Can you work these out from the model? Positions are in its coordinate system, mm. A direction names the side the tool comes from. Round coordinates to 2 decimals unless told otherwise and drop trailing zeros.
```python
from build123d import *

# Parameters (mm, degrees)
ESBO_O1_W             = 8
ESBO_O1_H             = 8
CORTE_EXTRUS_O1_DEPTH = 46
ESBO_O3_R             = 2.5
CORTE_EXTRUS_O2_DEPTH = 123.5


with BuildPart() as part:
    # Sketch1 → Revolve1 (revolve)
    with BuildSketch(Plane.XY):
        with BuildLine():
            Line((0, -20), (0, -122))
            ThreePointArc((0, -122), (0.146446609, -122.353553391), (0.5, -122.5))
            Line((0.5, -122.5), (9.616336506, -122.5))
            ThreePointArc((9.616336506, -122.5), (9.920717221, -122.39667667), (10.099299419, -122.129409523))
            Line((10.099299419, -122.129409523), (12.679491924, -112.5))
            Line((12.679491924, -112.5), (22.320508076, -112.5))
            Line((22.320508076, -112.5), (24.900700581, -122.129409523))
            ThreePointArc((24.900700581, -122.129409523), (25.079282779, -122.39667667), (25.383663494, -122.5))
            Line((25.383663494, -122.5), (34.5, -122.5))
            ThreePointArc((34.5, -122.5), (34.853553391, -122.353553391), (35, -122))
            Line((35, -122), (35, -50))
            Line((35, -50), (44.5, -50))
            ThreePointArc((44.5, -50), (44.853553391, -49.853553391), (45, -49.5))
            Line((45, -49.5), (45, -10))
            Line((45, -10), (2.5, -10))
            Line((2.5, -10), (0, -20))
        make_face()
    revolve(axis=Axis((0, 0, 0), (1, 0, 0)))

    # Esboço1 → Corte-extrusão1 (cut, through all)
    with BuildSketch(Plane.ZY):
        with Locations((0, -10)):
            Rectangle(ESBO_O1_W, ESBO_O1_H)
    extrude(amount=-CORTE_EXTRUS_O1_DEPTH, mode=Mode.SUBTRACT)

    # Esboço3 → Corte-extrusão2 (cut, through all)
    with BuildSketch(Plane.XY):
        with Locations((40, 0)):
            Circle(ESBO_O3_R)
    extrude(amount=-CORTE_EXTRUS_O2_DEPTH, mode=Mode.SUBTRACT)


solid = part.part
```
(1) Which directions (+Z, -Z, +X, -X, +Y, -Y) give clear straight access to the entire face, cutting with the end or side of a thin tool? Please do faces 1 (the cylindrical face through (23, 10, 0)), 2 (the conical face through (12.554, 24.489, 110.281)), 3 (the flat face through (35, 2, 53)).
(2) We'd pull the mould along Z, two halves only. Please class faces 4 (the conical face through (2.344, 8.432, 6.465)), 5 (the cylindrical face through (30.006, 26.556, 119.587)), 6 (the flat face through (23, -14, 0)), 7 (the flat face through (0, -2, 25)): released by +Z, released by -Z, zero draft, split by the parting line, or undercut.
(3) For pin 1 (8 mm diameter, centred on x = 18.5, z = 47, fed in from +Y); pin 2 (5 mm diameter, centred on x = 33.5, z = -32, fed in from -Y); pin 3 (4 mm diameter, centred on x = 23.5, z = 0, fed in from +Y); pin 4 (1 mm diameter, centred on x = 8.5, z = -96.5, fed in from -Y), each with a flat end and sliding along its axis, tell me the tip position at first contact or that it passes through.
(4) If I drill on line 1 (X direction, y = 0, z = -20); line 2 (Z direction, x = 30, y = 0); line 3 (Y direction, x = 17.5, z = 0), over which ranges is the centre line in solid material (lowest first)?
Check result:
1. face 1: +X, -X
1. face 2: none
1. face 3: +X
2. face 4: undercut
2. face 5: split by the parting line
2. face 6: undercut
2. face 7: zero draft
3. pin 1: stops at y = 103.96
3. pin 2: stops at y = -118.89
3. pin 3: stops at y = 122.5
3. pin 4: stops at y = -76.09
4. line 1: x = 0 to 37.5, 42.5 to 45
4. line 2: z = -122.5 to -10, 10 to 122.5
4. line 3: y = -112.5 to -14, 10 to 112.5
